Model file for the job. Use its own axes, mm. Face numbers are marked on the shaded views. A direction names the side the tool comes from. Round coordinates to 2 decimals unless told otherwise and drop trailing zeros. Order: outer loops, then holes, each group sorted by start corner. A loop starts at its lowest first (then second) coordinate and runs counter-clockwise, first axis right, second up. Notation, with made-up numbers: M -18,-18.5 L 7,-18.5 A21 ccw 7,5.5 Z; hole C 68,74.5 d8. An arc over 180 degrees is marked long. Return JSON: item names as keys, results as strings. Group by question number.
Item 1: Slice it at D-D on y = 14.5. Write the cut outline in (x, z).
Item 2: Which spindle directions (+Z, -Z, +X, -X, +Y, -Y) get a long thin tool onto all of the face, cutting with end or side? Do the marked faces 4, 5, 6 and 7. Say none if no direction does.
Item 3: Probe line 1 along Y through (x, z) = (10.5, 2.2); line 2 along X through (y, z) = (14.5, 6.5); line 3 along Z through (x, y) = (3.5, 20.25). List the from-to ranges inside material, lowest first.
Item 4: Pull direction X, two halves, no side cores. Call the marked faces 1, 2 and 3: pulls with the +X half, pulls with the -X half, needs draft (parallel to the pull), parting line crosses it, or undercut.
Item 5: Pin check, flat tips, straight feed: pin 1 Ø6.5 at (x, z) = (-2, 6) entering from +Y; pin 2 Ø4 at (x, y) = (7.5, 6.5) entering from +Z; pin 3 Ø4 at (x, z) = (2, 7.5) entering from -Y; pin 4 Ø5 at (x, z) = (0.5, 8.5) entering from +Y. Stop position of each tip, or through.
Item 6: Slice it at B-B on x = 0. Write the cut outline in (y, z) (3 decimals), then the cut area to 3 significant figures.
Item 7: Slice it at C-C on y = 19. Write the cut outline in (x, z).
Item 8: Slice it at A-A on z = 2. Write the cut outline in (x, y).
Autodesk Inventor part; units mm, degrees
ref_plane "YZ Plane" through (0, 0, 0) normal (1, 0, 0) x (0, 1, 0)
ref_plane "XZ Plane" through (0, 0, 0) normal (0, 1, 0) x (-1, 0, 0)
ref_plane "XY Plane" through (0, 0, 0) normal (0, 0, 1) x (1, 0, 0)
sketch "Náčrt1" plane through (0, 0, 0) normal (0, 0, 1) x (1, 0, 0)
  line L0 (12.5, 2) -> (12.5, 21.862)
  line L1 (10.5, 23.862) -> (0, 23.862)
  circle A0 centre (10.5, 2) radius 1.1
  arc A1 (12.5, 3.2809) -> (9.2191, 0) centre (10.5, 2) ccw
  circle A2 centre (10.5, 14.5) radius 1.1
  arc A3 (12.5, 15.7809) -> (12.5, 13.2191) centre (10.5, 14.5) ccw
  line L2 (0, 0) -> (10.5, 0)
  arc A4 (10.5, 0) -> (12.5, 2) centre (10.5, 2) ccw
  arc A5 (12.5, 21.862) -> (10.5, 23.862) centre (10.5, 21.862) ccw
  line L3 (-12.5, 2) -> (-12.5, 21.862)
  line L4 (-10.5, 23.862) -> (0, 23.862)
  circle A6 centre (-10.5, 2) radius 1.1
  arc A7 (-9.2191, 0) -> (-12.5, 3.2809) centre (-10.5, 2) ccw
  circle A8 centre (-10.5, 14.5) radius 1.1
  arc A9 (-12.5, 13.2191) -> (-12.5, 15.7809) centre (-10.5, 14.5) ccw
  line L5 (0, 0) -> (-10.5, 0)
  arc A10 (-12.5, 2) -> (-10.5, 0) centre (-10.5, 2) ccw
  arc A11 (-10.5, 23.862) -> (-12.5, 21.862) centre (-10.5, 21.862) ccw
  dimension "d2" = 2.2
  dimension "d3" = 2
  dimension "d6" = 2.2
  dimension "d8" = 4.75
  dimension "d9" = 2
  dimension "d10" = 23.862
  dimension "d11" = 2
extrude "Vysunutí1" add sketch "Náčrt1" along normal blind 3
sketch "Náčrt2" plane through (0, 0, 3) normal (0, 0, 1) x (1, 0, 0)
  line L0 (0, 0) -> (0, 23.862)
  line L1 (10.5, 23.862) -> (-10.5, 23.862)
  arc A0 (0, 11.525) -> (0, 17.275) centre (0, 14.4) ccw
  line L2 (-10.5, 0) -> (10.5, 0)
  line L3 (-5.4, 9) -> (5.4, 9)
  line L4 (5.4, 9) -> (5.4, 19.8)
  line L5 (5.4, 19.8) -> (-5.4, 19.8)
  line L6 (-5.4, 19.8) -> (-5.4, 9)
  line L7 (-5.4, 9) -> (5.4, 19.8) construction
  line L8 (5.4, 9) -> (-5.4, 19.8) construction
  arc A1 (0, 17.275) -> (0, 11.525) centre (0, 14.4) ccw
  dimension "d14" = 2.875
  dimension "d15" = 14.4
  dimension "d16" = 10.8
  dimension "d17" = 10.8
extrude "Vysunutí2" add sketch "Náčrt2" along normal blind 8 contours A0 L0 L5 L4 L3 | L0 L3 L6 L5 A1
properties part number "kamera"
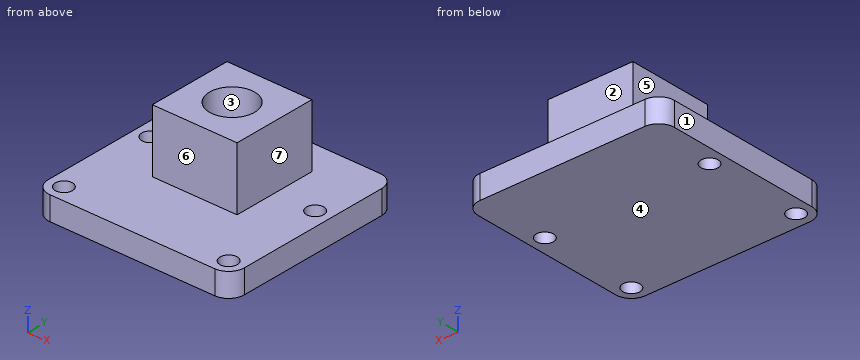
Output values:
{
 "1": {"outline": "M -12.5,0 L -11.6,0 L -11.6,3 L -12.5,3 Z; M -9.4,0 L 9.4,0 L 9.4,3 L 5.4,3 L 5.4,11 L 2.87,11 L 2.87,3 L -2.87,3 L -2.87,11 L -5.4,11 L -5.4,3 L -9.4,3 Z; M 11.6,0 L 12.5,0 L 12.5,3 L 11.6,3 Z"},
 "2": {"face 4": "-Z, +X, -X, +Y, -Y", "face 5": "+Z, -X, +Y, -Y", "face 6": "+Z, +X, -X, -Y", "face 7": "+Z, +X, +Y, -Y"},
 "3": {"line 1": "0 to 0.9, 3.1 to 13.4, 15.6 to 23.86", "line 2": "-5.4 to -2.87, 2.87 to 5.4", "line 3": "0 to 3"},
 "4": {"face 1": "pulls with the -X half", "face 2": "needs draft", "face 3": "undercut"},
 "5": {"pin 1": "y = 23.86", "pin 2": "z = 3", "pin 3": "y = 9", "pin 4": "y = 19.8"},
 "6": {"outline": "M 0,0 L 23.862,0 L 23.862,3 L 19.8,3 L 19.8,11 L 17.275,11 L 17.275,3 L 11.525,3 L 11.525,11 L 9,11 L 9,3 L 0,3 Z", "area": "112 mm²"},
 "7": {"outline": "M -12.5,0 L 12.5,0 L 12.5,3 L 5.4,3 L 5.4,11 L -5.4,11 L -5.4,3 L -12.5,3 Z"},
 "8": {"outline": "M -12.5,2 A2 ccw -10.5,0 L 10.5,0 A2 ccw 12.5,2 L 12.5,21.86 A2 ccw 10.5,23.86 L -10.5,23.86 A2 ccw -12.5,21.86 Z; hole C -10.5,2 d2.2; hole C -10.5,14.5 d2.2; hole C 10.5,2 d2.2; hole C 10.5,14.5 d2.2"}
}
